For this review, use the dimensioned drawing (mm, ordinates from the lowest corner) and the shaded views. Round coordinates to 2 decimals unless told otherwise and drop trailing zeros. Write each question's results on one line, items separated by ' | '. Start each with the question number.
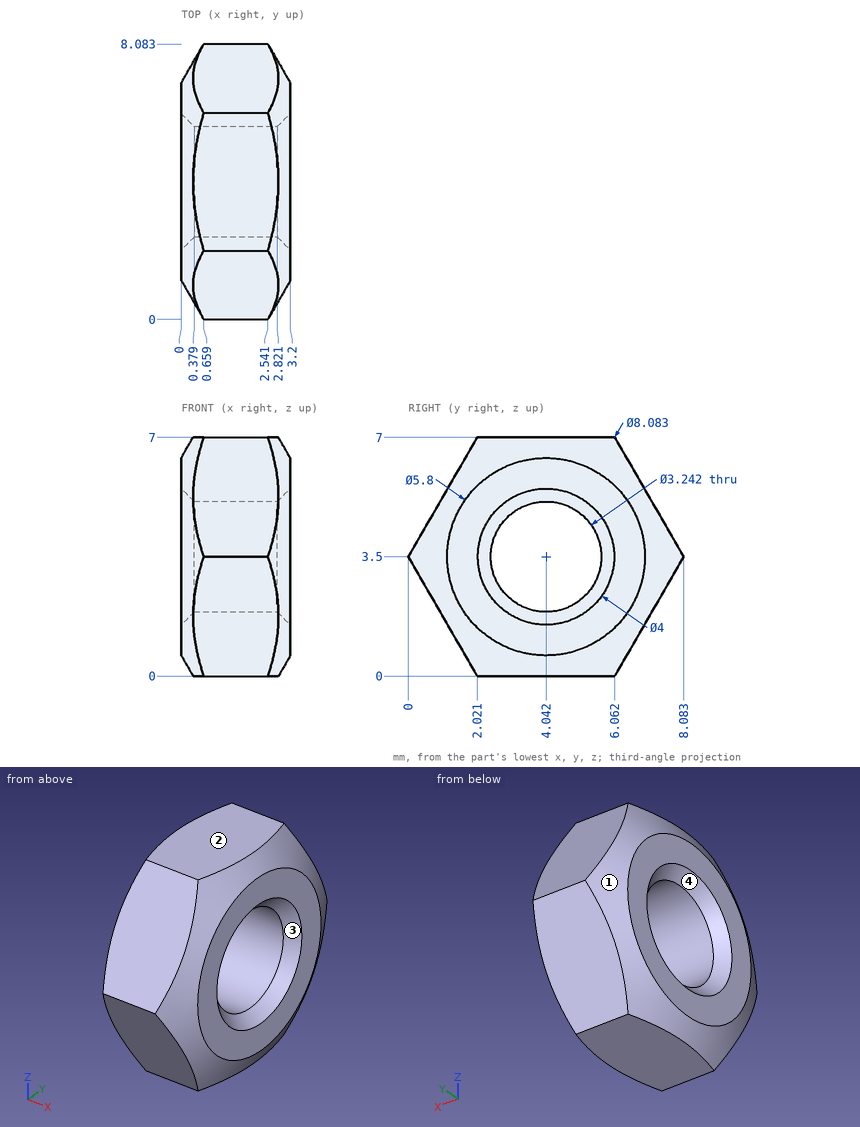
1) To check wall thickness, follow line 1 (Z direction, x = 2.75, y = 4); line 2 (Z direction, x = 2.45, y = 5.5) (1 decimal); line 3 (Y direction, x = 2.25, z = 4.5) (1 decimal). State the ranges of each line that lie inside material, in increasing order. Write a range as from..to.
2) Insertion check: pin 1 (1 mm diameter, centred on x = 1, y = 7, fed in from -Z); pin 2 (1.5 mm diameter, centred on x = 2, z = 3, fed in from +Y); pin 3 (1 mm diameter, centred on y = 1, z = 1, fed in from -X). Each pin has a flat end and moves straight along its axis. Give the tip position at first contact, or say it passes through.
3) The part is to be moulded in two halves that separate along Z. For the marked faces 1, 2, 3 and 4, say which applies: +Z half, -Z half, draft (parallel to the pull), parting line (faces both ways), or undercut.
Geometry check:
1) line 1: z = 0..1.88, 5.12..7 | line 2: z = 0..2.8, 4.2..7 | line 3: y = 0.6..2.8, 5.3..7.5
2) pin 1: stops at z = 0.76 | pin 2: stops at y = 8.08 | pin 3: stops at x = 0.31
3) face 1: parting line | face 2: +Z half | face 3: undercut | face 4: undercut
